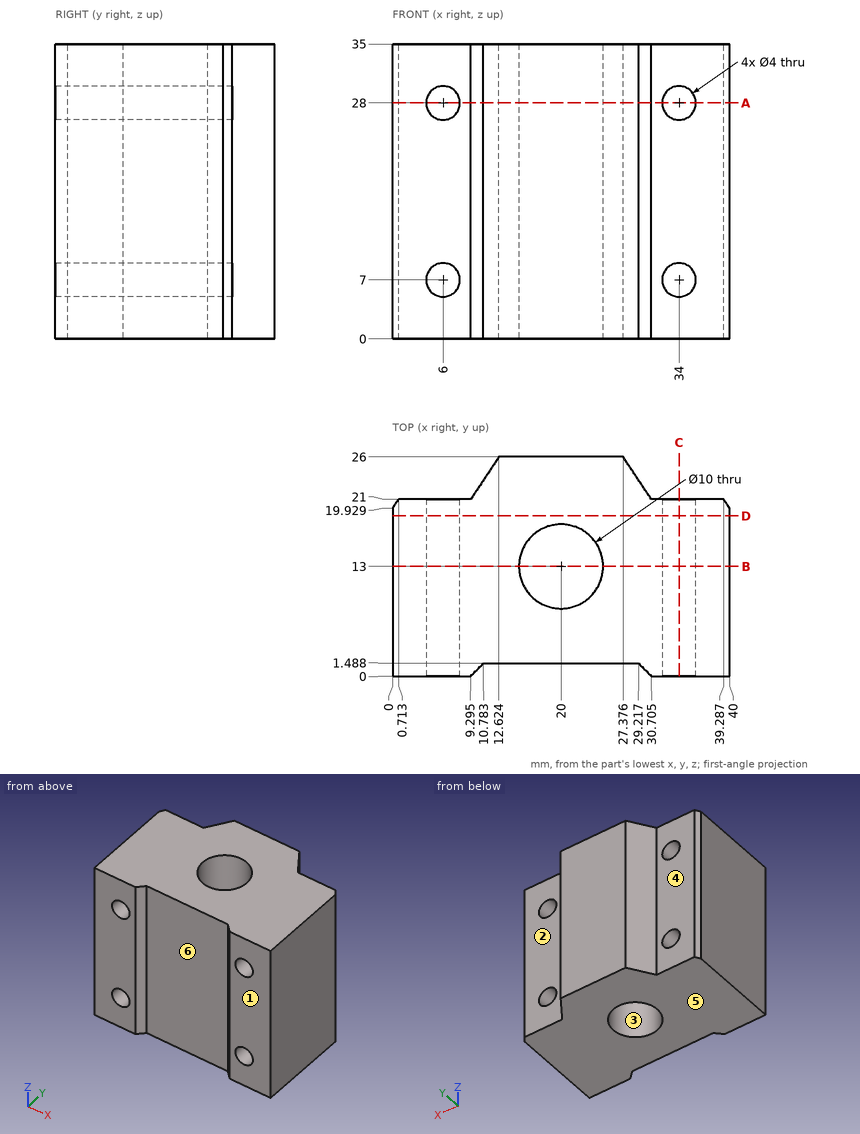
Check sheet for the drawn part. Datum: minimum x, y, z corner. Units: mm. A direction names the side the tool comes from. Round coordinates to 2 decimals unless told otherwise and drop trailing zeros. Loops run counter-clockwise (first coordinate to the right, second up) from the corner with the lowest first, then second, coordinate; pieces in that order, holes last. Notation, with made-up numbers: (33, -22.5) - (80, -22.5) arc R31 ccw to (80, 13.5) - close; hole circle Ø1 at (54.25, 26.25). An arc over 180 degrees is marked (long way). Write item = value, one per line. Start each with the question number.
1. Section check C-C on x = 34. Enter the section's corners in (y, z), then the cut area to 3 significant figures.
2. Section check A-A on z = 28. Enter the section's corners in (x, y) (1 decimal).
3. Section check B-B on y = 13. Enter the section's corners in (x, z), then the cut area to 4 significant figures.
4. Section check D-D on y = 19. Enter the section's corners in (x, z), then the cut area to 3 significant figures.
5. Set-up check for the marked faces 4, 5 and 6: record each of +Z, -Z, +X, -X, +Y, -Y from which the full face is reachable in a straight line by a thin tool's end or side.
6. Thickness scan on line 1 (Z direction, x = 6, y = 9.5); line 2 (Z direction, x = 32.5, y = 20.25) (1 decimal); line 3 (X direction, y = 13.25, z = 10). Record the ranges inside material, lowest first.
7. Mould release check, pull along Y, two halves, no side actions. Record for the marked faces 1, 2 and 3: released by +Y, released by -Y, zero draft, split by the parting line, or undercut.
8. Depth check by flat-ended pin: pin 1 (9 mm diameter, centred on x = 20, y = 13, fed in from -Z); pin 2 (5 mm diameter, centred on x = 17, z = 28.5, fed in from -Y); pin 3 (6 mm diameter, centred on x = 27, z = 20, fed in from -Y) (1 decimal); pin 4 (4.5 mm diameter, centred on x = 34, z = 7, fed in from +Y). Enter the tip coordinate at first touch or a pass-through.
Working result:
q1.outline = (0, 0) - (21, 0) - (21, 5) - (0, 5) - close; (0, 9) - (21, 9) - (21, 26) - (0, 26) - close; (0, 30) - (21, 30) - (21, 35) - (0, 35) - close
q1.area = 567 mm^2
q2.outline = (0, 0) - (4, 0) - (4, 21) - (0.7, 21) - (0, 19.9) - close; (8, 0) - (9.3, 0) - (10.8, 1.5) - (29.2, 1.5) - (30.7, 0) - (32, 0) - (32, 21) - (30.7, 21) - (27.4, 26) - (12.6, 26) - (9.3, 21) - (8, 21) - close; (36, 0) - (40, 0) - (40, 19.9) - (39.3, 21) - (36, 21) - close; hole circle Ø10 at (20, 13)
q3.outline = (0, 0) - (15, 0) - (15, 35) - (0, 35) - close; (25, 0) - (40, 0) - (40, 35) - (25, 35) - close; hole circle Ø4 at (6, 7); hole circle Ø4 at (6, 28); hole circle Ø4 at (34, 7); hole circle Ø4 at (34, 28)
q3.area = 1,000 mm^2
q4.outline = (0, 0) - (40, 0) - (40, 35) - (0, 35) - close; hole circle Ø4 at (6, 7); hole circle Ø4 at (6, 28); hole circle Ø4 at (34, 7); hole circle Ø4 at (34, 28)
q4.area = 1,350 mm^2
q5.face_4 = +Z, -Z, -X, +Y
q5.face_5 = -Z, +X, -X, +Y, -Y
q5.face_6 = +Z, -Z, -Y
q6.line_1 = 0 to 5, 9 to 26, 30 to 35
q6.line_2 = 0 to 5.7, 8.3 to 26.7, 29.3 to 35
q6.line_3 = 0 to 15.01, 24.99 to 40
q7.face_1 = released by -Y
q7.face_2 = released by +Y
q7.face_3 = undercut
q8.pin_1 = through
q8.pin_2 = 1.49
q8.pin_3 = 0.7
q8.pin_4 = 21
